Design review of the part built by this model. Coordinates are the model's own, in mm. A direction names the side the tool comes from. Coordinates: 2 decimals unless noted, no trailing zeros. Write each loop counter-clockwise with the first axis right and the second up, starting at its lowest first coordinate (ties: lowest second). Pieces come first, ordered by that corner, then holes. Notation, with made-up numbers: M 36.5,89.25 L 64.5,89.25 A28 cw 64.5,117.25 Z; hole C 17,-35.5 d8. An arc over 180 degrees is marked long. One line per question, with ' | ' between items.
from build123d import *

# Parameters (mm, degrees)
EXTRUDE_1_DEPTH     = 17.5
SKETCH_2_W          = 35.2
SKETCH_2_H          = 27.5
CUT_EXTRUDE_1_DEPTH = 35.2
CUT_EXTRUDE_2_DEPTH = 60.213596412
CUT_EXTRUDE_3_DEPTH = 60.213596412
SKETCH_5_W          = 34
SKETCH_5_H          = 6.2
SKETCH_5_W_2        = 28
SKETCH_5_H_2        = 10
CUT_EXTRUDE_4_DEPTH = 3.2
SKETCH_6_W          = 34
SKETCH_6_H          = 6.2
SKETCH_6_W_2        = 28
SKETCH_6_H_2        = 10
CUT_EXTRUDE_5_DEPTH = 3.2
FILLET_1_R          = 2


with BuildPart() as part:
    # Эскиз1 → Бобышка-Вытянуть1 (new, symmetric)
    with BuildSketch(Plane(origin=(0, 0, 0), x_dir=(1, 0, 0), z_dir=(0, 1, 0))):
        with BuildLine():
            Line((0, 40), (0, 0))
            Line((0, 0), (40, 0))
            Line((40, 0), (40, 5.3))
            ThreePointArc((40, 5.3), (39.414213562, 6.714213562), (38, 7.3))
            Line((38, 7.3), (32, 7.3))
            Line((32, 7.3), (7.3, 32))
            Line((7.3, 32), (7.3, 38))
            ThreePointArc((7.3, 38), (6.714213562, 39.414213562), (5.3, 40))
            Line((5.3, 40), (0, 40))
        make_face()
    extrude(amount=EXTRUDE_1_DEPTH, both=True)

    # Эскиз2 → Вырез-Вытянуть1 (cut)
    with BuildSketch(Plane(origin=(0, 0, -40), x_dir=(-1, 0, 0), z_dir=(0, 0, -1))):
        with Locations((-22.4, 0)):
            Rectangle(SKETCH_2_W, SKETCH_2_H)
    extrude(amount=-CUT_EXTRUDE_1_DEPTH, mode=Mode.SUBTRACT)

    # Эскиз3 → Вырез-Вытянуть2 (cut, through all)
    with BuildSketch(Plane.XY):
        with BuildLine():
            Line((13.5, 4.55), (27.5, 4.55))
            ThreePointArc((27.5, 4.55), (32.05, 0), (27.5, -4.55))
            Line((27.5, -4.55), (13.5, -4.55))
            ThreePointArc((13.5, -4.55), (8.95, 0), (13.5, 4.55))
        make_face()
    extrude(amount=-CUT_EXTRUDE_2_DEPTH, mode=Mode.SUBTRACT)

    # Эскиз4 → Вырез-Вытянуть3 (cut, through all)
    with BuildSketch(Plane.ZY):
        with BuildLine():
            Line((-27.5, 4.55), (-13.5, 4.55))
            ThreePointArc((-13.5, 4.55), (-8.95, 0), (-13.5, -4.55))
            Line((-13.5, -4.55), (-27.5, -4.55))
            ThreePointArc((-27.5, -4.55), (-32.05, 0), (-27.5, 4.55))
        make_face()
    extrude(amount=-CUT_EXTRUDE_3_DEPTH, mode=Mode.SUBTRACT)

    # Эскиз5 → Вырез-Вытянуть4 (cut)
    with BuildSketch(Plane.ZY):
        with Locations((-20, 11)):
            Rectangle(SKETCH_5_W, SKETCH_5_H)
        with Locations((-20, -11)):
            Rectangle(SKETCH_5_W, SKETCH_5_H)
        with Locations((-20, 0)):
            Rectangle(SKETCH_5_W_2, SKETCH_5_H_2)
    extrude(amount=-CUT_EXTRUDE_4_DEPTH, mode=Mode.SUBTRACT)

    # Эскиз6 → Вырез-Вытянуть5 (cut)
    with BuildSketch(Plane.XY):
        with Locations((20, 11)):
            Rectangle(SKETCH_6_W, SKETCH_6_H)
        with Locations((20, -11)):
            Rectangle(SKETCH_6_W, SKETCH_6_H)
        with Locations((20, 0)):
            Rectangle(SKETCH_6_W_2, SKETCH_6_H_2)
    extrude(amount=-CUT_EXTRUDE_5_DEPTH, mode=Mode.SUBTRACT)

    # Скругление1
    fillet_1_edges = [part.edges().sort_by_distance(p)[0] for p in [
        (7.3, 15.625, -32),
        (32, 15.625, -7.3),
        (7.3, -15.625, -32),
        (32, -15.625, -7.3),
    ]]
    fillet(fillet_1_edges, radius=FILLET_1_R)


solid = part.part
1. Take a section at A-A (y = 12.5). Write out the cut boundary in (x, z), then the cut area to 3 significant figures.
Answer sheet:
outline: M 0,-40 L 4.8,-40 L 4.8,-4.8 L 40,-4.8 L 40,0 L 37,0 L 37,-3.2 L 3.2,-3.2 L 3.2,-37 L 0,-37 Z; M 0,-3 L 3,-3 L 3,0 L 0,0 Z | area: 143 mm^2
2. Take a section at D-D (y = 0). Write out the cut boundary in (x, z).
Answer sheet:
outline: M 0,-40 L 4.8,-40 L 4.8,-32.05 L 3.2,-32.05 L 3.2,-34 L 0,-34 Z; M 0,-6 L 3.2,-6 L 3.2,-8.95 L 4.8,-8.95 L 4.8,-4.8 L 8.95,-4.8 L 8.95,-3.2 L 6,-3.2 L 6,0 L 0,0 Z; M 32.05,-4.8 L 40,-4.8 L 40,0 L 34,0 L 34,-3.2 L 32.05,-3.2 Z
3. Tool access review of faces 1 (the face through (20, -11, -3.2)), 2 (the face through (2, 0, -34)), 3 (the face through (6, 0, -2)), 4 (the face through (4, -4.55, -20)): name each direction out of +Z, -Z, +X, -X, +Y, -Y from which nothing blocks a thin tool from reaching the whole face with its end or side.
Answer sheet:
face 1: +Z, -X | face 2: -X | face 3: +Z | face 4: +X, -X
4. Insertion check: pin 1 Ø1.9 at (y, z) = (-11, -20) entering from -X; pin 2 Ø3 at (x, y) = (23, 11) entering from +Z; pin 3 Ø1.1 at (x, y) = (34.5, 15) entering from -Z; pin 4 Ø6 at (x, z) = (34.5, -12) entering from +Y. Each pin has a flat end and moves straight along its axis. Give the tip position at first contact, or say it passes through.
Answer sheet:
pin 1: x = 3.2 | pin 2: z = -3.2 | pin 3: z = -7.3 | pin 4: through
5. To check wall thickness, follow line 1 along Y through (x, z) = (3, -13.5); line 2 along Y through (x, z) = (4.5, -17.5); line 3 along Y through (x, z) = (8.5, -10.5). State the ranges of each line that lie inside material, in increasing order. Write a range as [from, to].
Answer sheet:
line 1: [-17.5, -14.1], [-7.9, -5], [5, 7.9], [14.1, 17.5] | line 2: [-17.5, -4.55], [4.55, 17.5] | line 3: [-17.5, -13.75], [13.75, 17.5]
6. Draft analysis for pull direction Z (two halves, no side actions). For faces 5 (the face through (6.73, 15.65, -39.4)), 6 (the face through (2, 5, -20)), 7 (the face through (37, 11, -2)), state which applies: pulls with the +Z half, pulls with the -Z half, needs draft (parallel to the pull), parting line crosses it, or undercut.
Answer sheet:
face 5: pulls with the -Z half | face 6: undercut | face 7: needs draft
7. Take a section at C-C (x = 35). Write out the cut boundary in (y, z).
Answer sheet:
outline: M -17.5,-7.3 L -13.75,-7.3 L -13.75,-4.8 L 13.75,-4.8 L 13.75,-7.3 L 17.5,-7.3 L 17.5,0 L 14.1,0 L 14.1,-3.2 L 7.9,-3.2 L 7.9,0 L -7.9,0 L -7.9,-3.2 L -14.1,-3.2 L -14.1,0 L -17.5,0 Z
8. Take a section at B-B (z = -35). Write out the cut boundary in (x, y).
Answer sheet:
outline: M 0,-17.5 L 7.3,-17.5 L 7.3,-13.75 L 4.8,-13.75 L 4.8,13.75 L 7.3,13.75 L 7.3,17.5 L 0,17.5 L 0,14.1 L 3.2,14.1 L 3.2,7.9 L 0,7.9 L 0,-7.9 L 3.2,-7.9 L 3.2,-14.1 L 0,-14.1 Z
